Can you work these out from the model? Positions are in its coordinate system, mm. A direction names the side the tool comes from. Give positions to 0.01 mm unless a question says otherwise; leave off trailing zeros. Write each loop counter-clockwise with the first axis right and the second up, starting at its lowest first coordinate (ties: lowest second). Pieces come first, ordered by that corner, then holes.
Autodesk Inventor part; units mm, degrees
ref_plane "YZ Plane" through (0, 0, 0) normal (1, 0, 0) x (0, 1, 0)
ref_plane "XZ Plane" through (0, 0, 0) normal (0, 1, 0) x (-1, 0, 0)
ref_plane "XY Plane" through (0, 0, 0) normal (0, 0, 1) x (1, 0, 0)
sketch "Sketch1" plane through (0, 0, 0) normal (0, 1, 0) x (-1, 0, 0)
  line L0 (0, 0) -> (-40, 0)
  line L1 (-40, 0) -> (-40, -2)
  line L2 (-40, -2) -> (0, -2)
  line L3 (0, -2) -> (0, 0)
  dimension "d0" = 40
  dimension "d1" = 2
extrude "Extrusion1" add sketch "Sketch1" along normal blind 44
sketch "Sketch2" plane through (0, 0, 0) normal (0, 0, 1) x (1, 0, 0)
  line L0 (40, 44) -> (0, 44) construction
  line L1 (0, 44) -> (40, 0) construction
  line L2 (40, 44) -> (0, 0) construction
  circle A0 centre (20, 22) radius 6.75
  dimension "d4" = 13.5
extrude "Extrusion2" cut sketch "Sketch2" against normal blind 40
sketch "Sketch3" plane through (40, 0, -2) normal (0, 0, -1) x (-1, 0, 0)
  circle A0 centre (20, 22) radius 6.75 construction
  circle A1 centre (20, 22) radius 8.5 construction
  circle A2 centre (12.6388, 26.25) radius 1.1 construction
  circle A3 centre (27.3612, 26.25) radius 1.1 construction
  line L0 (20, 22) -> (27.3612, 26.25) construction
  line L1 (20, 22) -> (12.6388, 26.25) construction
  circle A4 centre (20, 13.5) radius 1.1 construction
  line L2 (20, 22) -> (20, 13.5) construction
  line L3 (40, 0) -> (40, 44) construction
  dimension "d7" = 17
  dimension "d9" = 2.2
  dimension "d10" = 2.2
  dimension "d22" = 2.2
  dimension "d25" = 120
  dimension "d26" = 120
hole "Hole1" at (20, 13.5, -2) at (12.6388, 26.25, -2) at (27.3612, 26.25, -2) direction (0, 0, 1) diameter 3.1 depth 8.8 tip angle 118
sketch "Sketch4" plane through (40, 0, 0) normal (1, 0, 0) x (0, 0, -1)
  line L0 (0, 44) -> (2, 44)
  line L1 (0, 0) -> (2, 0)
  line L2 (2, 0) -> (2, 44)
  line L3 (2, 44) -> (0, 44)
  line L4 (0, 44) -> (0, 0)
extrude "Extrusion3" add sketch "Sketch4" along normal blind 20
sketch "Sketch5" plane through (0, 0, -2) normal (0, 0, -1) x (-1, 0, 0)
  circle A0 centre (-44.75, 22) radius 13.2
  line L0 (0, 0) -> (-60, 0)
  line L1 (-60, 0) -> (-60.0955, 41.9998)
  line L2 (0, 0) -> (0, 44)
  dimension "d27" = 26.4
  dimension "d28" = 22
  dimension "d29" = 15.3
  dimension "d45" = 44.75
extrude "Extrusion4" cut sketch "Sketch5" against normal through all
sketch "Sketch6" plane through (60, 0, 0) normal (1, 0, 0) x (0, 0, -1)
  line L0 (0, 0) -> (0, 44)
  line L1 (2, 0) -> (0, 0)
  line L2 (0, 44) -> (2, 44)
  line L3 (2, 44) -> (2, 0)
  line L4 (2, 0) -> (0, 0)
  line L5 (0, 0) -> (0, 44)
extrude "Extrusion5" add sketch "Sketch6" along normal blind 34
fillet "Fillet1" radius 2 4 edges at (0, 44, -1) (0, 0, -1) (94, 44, -1) (94, 0, -1)
sketch "Sketch7" plane through (2, 0, 0) normal (0, 0, 1) x (1, 0, 0)
  circle A0 centre (87, 22) radius 2.5
  circle A1 centre (3, 22) radius 2.5
  line L0 (0, 44) -> (90, 44)
  line L1 (92, 42) -> (92, 2)
  line L2 (0, 0) -> (90, 0)
  line L3 (-2, 2) -> (-2, 42)
  circle A2 centre (87, 4) radius 2.5
  circle A3 centre (3, 4) radius 2.5
  point P0 (-2, 0)
  dimension "d53" = 5
  dimension "d54" = 5
  dimension "d55" = 22
  dimension "d56" = 5
  dimension "d57" = 22
  dimension "d58" = 5
  dimension "d69" = 44
  dimension "d73" = 5
  dimension "d74" = 18
  dimension "d75" = 5
hole "Hole2" at (5, 22, 0) at (89, 22, 0) at (89, 4, 0) at (5, 4, 0) direction (0, 0, -1) diameter 5 depth 14.2 tip angle 118
chamfer "Chamfer1" distance 0.3 angle 45 2 edges at (5, 24.5, -2) (89, 24.5, -2)
sketch "Sketch8" plane through (92, 0, -2) normal (0, 0, -1) x (-1, 0, 0)
  circle A0 centre (72, 22) radius 6.75
  circle A1 centre (72, 22) radius 6.75
  circle A2 centre (72, 22) radius 5.5
  point P0 (92, 0)
  dimension "d70" = 11
extrude "Extrusion6" add sketch "Sketch8" against normal blind 0.6
sketch "Sketch9" plane through (2, 0, 0) normal (0, 0, 1) x (1, 0, 0)
  circle A0 centre (58.5, 32.48) radius 1
  circle A1 centre (58.5, 11.52) radius 1
  line L0 (0, 44) -> (90, 44)
  line L1 (0, 0) -> (90, 0)
  line L2 (92, 42) -> (92, 2)
  point P0 (-2, 0)
  dimension "d76" = 2
  dimension "d77" = 2
  dimension "d78" = 20.96
  dimension "d79" = 44
  dimension "d80" = 11.52
  dimension "d81" = 33.5
hole "Hole3" at (60.5, 11.52, 0) at (60.5, 32.48, 0) direction (0, 0, -1) diameter 1.567 depth 6.3 tip angle 118
chamfer "Chamfer2" distance 0.2 angle 45 1 edges at (57.95, 22, 0)
chamfer "Chamfer3" distance 0.2 angle 45 2 edges at (60.5, 12.3035, 0) (60.5, 33.2635, 0)
sketch "Sketch10" plane through (2, 0, 0) normal (0, 0, 1) x (1, 0, 0)
  circle A0 centre (84.365, 34) radius 1
  circle A1 centre (74.365, 34) radius 1
  line L0 (0, 44) -> (90, 44)
  line L1 (92, 42) -> (92, 2)
  point P0 (-2, 0)
  dimension "d95" = 2
  dimension "d96" = 2
  dimension "d97" = 10
  dimension "d98" = 10
  dimension "d99" = 7.635
hole "Hole4" at (86.365, 34, 0) at (76.365, 34, 0) direction (0, 0, -1) diameter 2.459 depth 8.8 tip angle 118
chamfer "Chamfer4" distance 0.3 angle 45 2 edges at (86.365, 35.2295, 0) (76.365, 35.2295, 0)
equation "\"d55\" = 0.5 * d69"
equation "\"d57\" = 0.5 * d69"
equation "\"d80\" = -0.5 * d78 + 0.5 * d79"
properties part number "płyta silnika"
(1) For faces 1 (the face through (23.63, 27.69, -0.69)), 2 (the face through (54.5, 30.9, -1.1)), which set-ups out of +Z, -Z, +X, -X, +Y, -Y let a thin tool reach every point of the face, with its end or its side?
Returned:
face 1: +Z
face 2: +Z, -Z
(2) Imagine slicing it at D-D, the plane z = -0.85. Give the number of separate pieces and of enclosed holes in the cut face, plus the area to 3 significant figures.
Returned:
separate pieces: 1
enclosed holes: 13
area: 3,330 mm2
(3) Will these pins go through, and if not, where does the flat tip stop? P1, Ø10, axis at x = 52.5, y = 12, coming from the -Z side; P2, Ø3, axis at x = 76.365, y = 34, coming from the +Z side; P3, Ø1.9, axis at x = 20, y = 13.5, coming from the -Z side; P4, Ø1.8, axis at x = 60.5, y = 32.48, coming from the +Z side.
Returned:
P1: stops at z = -2
P2: stops at z = -0.03
P3: passes through
P4: stops at z = -0.08
(4) Imagine slicing it at C-C, the plane x = 5. Write out the boundary of the cut face in (y, z).
Returned:
outline: (0, -2) - (1.5, -2) - (1.5, 0) - (0, 0) - close; (6.5, -2) - (19.2, -2) - (19.5, -1.7) - (19.5, 0) - (6.5, 0) - close; (24.5, -1.7) - (24.8, -2) - (44, -2) - (44, 0) - (24.5, 0) - close
(5) If we mould it in two halves opening along Y, with no side actions, what happens to faces 3 (the face through (86.52, 22.33, -0.86)), 4 (the face through (87.11, 34.98, -1.16)), 5 (the face through (46, 44, -1)), 6 (the face through (58.1, 22.3, -2))? For each: +Y half, -Y half, draft (parallel to the pull), parting line (faces both ways), or undercut.
Returned:
face 3: undercut
face 4: undercut
face 5: +Y half
face 6: draft
(6) Imagine slicing it at B-B, the plane y = 4. Write out the boundary of the cut face in (x, z).
Returned:
outline: (0, -2) - (2.5, -2) - (2.5, 0) - (0, 0) - close; (7.5, -2) - (86.5, -2) - (86.5, 0) - (7.5, 0) - close; (91.5, -2) - (94, -2) - (94, 0) - (91.5, 0) - close
(7) Imagine slicing it at A-A, the plane x = 44.75. Write out the boundary of the cut face in (y, z), plus the area to 3 significant figures.
Returned:
outline: (0, -2) - (8.8, -2) - (8.8, -0.2) - (8.6, 0) - (0, 0) - close; (35.2, -2) - (44, -2) - (44, 0) - (35.4, 0) - (35.2, -0.2) - close
area: 35.2 mm2
(8) If I drill on L1, parallel to Y at x = 89, z = -0.5; L2, parallel to Y at x = 60.5, z = -1.3; L3, parallel to X at y = 4, z = -0.95, over which ranges is the centre line in solid material (lowest first)?
Returned:
L1: y = 0 to 1.5, 6.5 to 19.5, 24.5 to 44
L2: y = 0 to 10.74, 12.3 to 31.7, 33.26 to 44
L3: x = 0 to 2.5, 7.5 to 86.5, 91.5 to 94
